Read the model definition and answer for the solid it produces. Units are mm, in the model's axes. A direction names the side the tool comes from. Coordinates: 2 decimals unless noted, no trailing zeros. Write each loop counter-clockwise with the first axis right and the second up, starting at its lowest first coordinate (ties: lowest second). Pieces come first, ordered by that corner, then holes.
(1) Section C-C on x = -42 is taken. Write down the section's boundary in (y, z) (1 decimal), then the cut area to 3 significant figures.
(2) Section A-A on y = -73.5 is taken. Write down the section's boundary in (x, z) (3 decimals), then the cut area to 3 significant figures.
(3) Section D-D on y = -49 is taken. Write down the section's boundary in (x, z), then the cut area to 3 significant figures.
(4) Given pin 1 (1.5 mm diameter, centred on y = -69.5, z = 20.5, fed in from +X); pin 2 (1.5 mm diameter, centred on y = -4, z = 7, fed in from -X); pin 3 (5 mm diameter, centred on x = -77, z = -11.5, fed in from +Y), each flat-ended and moving along its own axis, determine where each tip first touches the part or whether it passes through.
(5) Find the intervals of material crossed by probe 1 along X at (y, z) = (2.5, 22); probe 2 along Z at (x, y) = (8.5, 9.5); probe 3 along Y at (x, z) = (-41, -8.5), in increasing order.
(6) Which of the six approach directions +Z, -Z, +X, -X, +Y, -Y give full straight-line access (tool end or side, diameter ignored) to faces 1 (the flat face through (-43, -98, -15.875)), 2 (the flat face through (-17.462, -1, 13)), 3 (the flat face through (0, -67.469, -8))?
(7) The mould has two halves that part along X. Classify faces 4 (the cylindrical face through (-40.698, -126.922, 5.051)), 5 (the cylindrical face through (-42.545, -92.006, 5.051)), 6 (the flat face through (-84, -67.469, 5)): +X half, -X half, draft (parallel to the pull), parting line (faces both ways), or undercut.
from build123d import *

# Parameters (mm, degrees)
F0_W     = 34.925
F0_H     = 134.9375
F1_DEPTH = 25.4
F2_DEPTH = 25.4
F4_DEPTH = 15.875


with BuildPart() as f1:
    # F0 (on Top) → F1 (new body)
    with BuildSketch(Plane.XY):
        Rectangle(F0_W, F0_H)
    extrude(amount=F1_DEPTH)

    # F0 (on Top) → F2 (join)
    with BuildSketch(Plane.XY):
        Rectangle(F0_W, F0_H)
        with BuildLine():
            Line((17.4625, -67.46875), (-17.4625, -67.46875))
            ThreePointArc((-17.4625, -67.46875), (-42.00525, -92.0115), (-66.548, -67.46875))
            Line((-66.548, -67.46875), (-101.473, -67.46875))
            ThreePointArc((-101.473, -67.46875), (-42.00525, -126.9365), (17.4625, -67.46875))
        make_face()
    extrude(amount=F2_DEPTH)

    # F3 (on face) → F4 (join)
    with BuildSketch(Plane(origin=(0, 0, 0), x_dir=(1, 0, 0), z_dir=(0, 0, -1))):
        with BuildLine():
            ThreePointArc((-66.548, 67.46875), (-42.00525, 92.0115), (-17.4625, 67.46875))
            Line((-17.4625, 67.46875), (17.4625, 67.46875))
            ThreePointArc((17.4625, 67.46875), (-42.00525, 126.9365), (-101.473, 67.46875))
            Line((-101.473, 67.46875), (-66.548, 67.46875))
        make_face()
    extrude(amount=F4_DEPTH)


solid = f1.part
Response:
1. outline: (-126.9, -15.9) - (-92, -15.9) - (-92, 25.4) - (-126.9, 25.4) - close
1. area: 1,440 mm2
2. outline: (-101.166, -15.875) - (-65.795, -15.875) - (-65.795, 25.4) - (-101.166, 25.4) - close; (-18.215, -15.875) - (17.156, -15.875) - (17.156, 25.4) - (-18.215, 25.4) - close
2. area: 2,920 mm2
3. outline: (-17.46, 0) - (17.46, 0) - (17.46, 25.4) - (-17.46, 25.4) - close
3. area: 887 mm2
4. pin 1: stops at x = 17.45
4. pin 2: stops at x = -17.46
4. pin 3: stops at y = -67.47
5. probe 1: x = -17.46 to 17.46
5. probe 2: z = 0 to 25.4
5. probe 3: y = -126.93 to -91.99
6. face 1: -Z, +X, -X, +Y, -Y
6. face 2: +Z, -Z, -X, +Y
6. face 3: -Z, +X, -X, +Y
7. face 4: parting line
7. face 5: undercut
7. face 6: draft
